from build123d import *

# Parameters (mm, degrees)
SKETCH1_W           = 6.6
SKETCH1_H           = 6.6
BOSS_EXTRUDE1_DEPTH = 2.5
CHAMFER1_SIZE       = 1
SKETCH3_R           = 3.5
CUT_EXTRUDE1_DEPTH  = 1
CUT_EXTRUDE3_DEPTH  = 1.399267399


with BuildPart() as part:
    # Sketch1 → Boss-Extrude1 (new body)
    with BuildSketch(Plane(origin=(0, 0, 0), x_dir=(1, 0, 0), z_dir=(0, 1, 0))):
        Rectangle(SKETCH1_W, SKETCH1_H)
    extrude(amount=BOSS_EXTRUDE1_DEPTH)

    # Chamfer1
    chamfer1_edges = [part.edges().sort_by_distance(p)[0] for p in [
        (3.3, 1.25, 3.3),
        (-3.3, 1.25, 3.3),
    ]]
    chamfer(chamfer1_edges, length=CHAMFER1_SIZE)

    # Sketch3 → Cut-Extrude1 (cut)
    with BuildSketch(Plane(origin=(0, 2.5, 0), x_dir=(1, 0, 0), z_dir=(0, 1, 0))):
        Circle(SKETCH3_R)
    extrude(amount=-CUT_EXTRUDE1_DEPTH, mode=Mode.SUBTRACT)

    # Sketch6 → Cut-Extrude3 (cut, through all)
    with BuildSketch(Plane(origin=(0, 0.19926807, -0.012076853), x_dir=(1, 0, 0), z_dir=(0, 0.998168497, -0.06049506))):
        with BuildLine():
            Line((-0.45, 3.293956039), (-0.45, 1.097985346))
            add(Edge.make_bspline(
                [(-0.45, 1.097985346), (-0.45, 0.648809523), (0, 0.648809523), (0.45, 0.648809523), (0.45, 1.097985346)],
                knots=[3.141592654, 3.141592654, 3.141592654, 4.71238898, 4.71238898, 6.283185307, 6.283185307, 6.283185307], degree=2, weights=[1, 0.707106781, 1, 0.707106781, 1]))
            Line((0.45, 1.097985346), (0.45, 3.293956039))
            Line((0.45, 3.293956039), (-0.45, 3.293956039))
        make_face()
    cut_extrude3 = extrude(amount=-CUT_EXTRUDE3_DEPTH, mode=Mode.SUBTRACT)

    # Mirror1: Cut-Extrude3 across plane
    add(cut_extrude3.mirror(Plane.XY), mode=Mode.SUBTRACT)


solid = part.part
Design review of the part built by this model. Coordinates are the model's own, in mm. A direction names the side the tool comes from. Round coordinates to 2 decimals unless told otherwise and drop trailing zeros. Loops run counter-clockwise (first coordinate to the right, second up) from the corner with the lowest first, then second, coordinate; pieces in that order, holes last. Notation, with made-up numbers: M 24.25,37.25 L 38.25,37.25 A14 cw 38.25,59.25 Z; hole C 82.5,69 d3. An arc over 180 degrees is marked long. Answer as a JSON object with one key per item and string values.
Item 1: We need section C-C on x = 1.5. Give the boundary of the cut face in (y, z).
Answer sheet:
{"outline": "M 0,-3.3 L 2.5,-3.3 L 2.5,-3.16 L 1.5,-3.16 L 1.5,3.16 L 2.5,3.16 L 2.5,3.3 L 0,3.3 Z"}
Item 2: Wall thickness on L1, parallel to Y at x = 1, z = -2; L2, parallel to Z at x = -2.75, y = 1.7; L3, parallel to X at y = 1.9, z = 1.75: over which ranges is each line inside the solid? List them lowest first. Write a range as from..to.
Answer sheet:
{"L1": "y = 0..1.5", "L2": "z = -3.3..-2.17, 2.17..2.85", "L3": "x = -3.3..-3.03, 3.03..3.3"}
Item 3: We need section D-D on y = 0.85. Give the boundary of the cut face in (x, z), and give its area (3 significant figures).
Answer sheet:
{"outline": "M -3.3,-3.3 L 3.3,-3.3 L 3.3,2.3 L 2.3,3.3 L -2.3,3.3 L -3.3,2.3 Z", "area": "42.6 mm^2"}
Item 4: Clearance check with a flat-ended pin moving along its axis: P1, Ø3.5, axis at x = 0, z = -1.5, coming from the +Y side. State where the tip first meets the part, or that it passes through.
Answer sheet:
{"P1": "stops at y = 1.5"}
Item 5: Machinability: for faces 4 (the cylindrical face through (-2.46, 2.01, -2.49)), 5 (the flat face through (-0.01, 0.08, 2)), 6 (the flat face through (3.3, 1, 0)), which of the approach directions +Z, -Z, +X, -X, +Y, -Y give a long, thin tool a straight path to every point of the face, cutting with its end or side? Answer none if there is none.
Answer sheet:
{"face 4": "+Y", "face 5": "-Y", "face 6": "+Z, -Z, +X, +Y, -Y"}
Item 6: We need section A-A on y = 1.8. Give the boundary of the cut face in (x, z).
Answer sheet:
{"outline": "M -3.3,-3.3 L -1.17,-3.3 A3.5 cw -3.3,-1.17 Z; M -3.3,1.17 A3.5 cw -1.17,3.3 L -2.3,3.3 L -3.3,2.3 Z; M 1.17,-3.3 L 3.3,-3.3 L 3.3,-1.17 A3.5 cw Z; M 1.17,3.3 A3.5 cw 3.3,1.17 L 3.3,2.3 L 2.3,3.3 Z"}
Item 7: The part is to be moulded in two halves that separate along X. For faces 1 (the flat face through (-3.3, 1, 0)), 2 (the flat face through (3, 2.5, -3)), 3 (the flat face through (0, 1.5, 0)), say which applies: pulls with the +X half, pulls with the -X half, needs draft (parallel to the pull), parting line crosses it, or undercut.
Answer sheet:
{"face 1": "pulls with the -X half", "face 2": "needs draft", "face 3": "undercut"}
